Check sheet for the modelled part. Datum: model origin and axes. Units: mm. Face numbers are marked on the shaded views. Round coordinates to 2 decimals unless told otherwise and drop trailing zeros. Order: outer loops, then holes, each group sorted by start corner. A loop starts at its lowest first (then second) coordinate and runs counter-clockwise, first axis right, second up. Notation, with made-up numbers: (2.25, 18) -> (57.25, 18) arc R23 cw to (57.25, 38) -> close; hole circle Ø7 at (21.25, -16.5). An arc over 180 degrees is marked (long way). Answer as CSV lines item,"result". Start each with the question number.
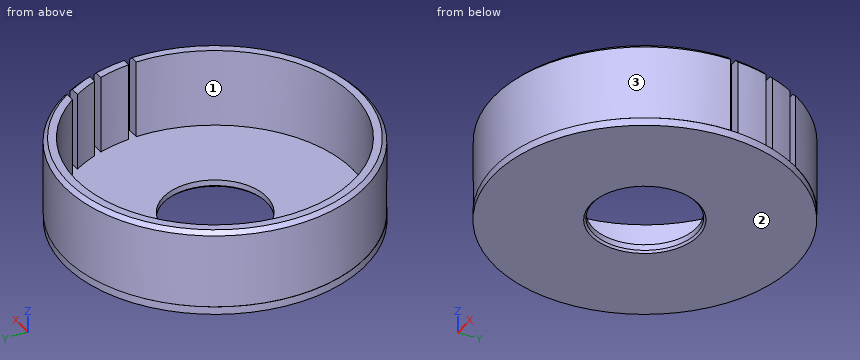
from build123d import *

# Parameters (mm, degrees)
SKETCH_R        = 38.5
SKETCH_R_2      = 13.2
PAD_DEPTH       = 2
PAD001_DEPTH    = 20
PAD002_DEPTH    = 20
PAD003_DEPTH    = 20
CHAMFER_SIZE    = 1
CHAMFER001_SIZE = 1
CHAMFER002_SIZE = 1
CHAMFER003_SIZE = 0.5


with BuildPart() as part:
    # Sketch → Pad (new body)
    with BuildSketch(Plane.XY):
        Circle(SKETCH_R)
        Circle(SKETCH_R_2, mode=Mode.SUBTRACT)
    extrude(amount=PAD_DEPTH)

    # Sketch001 (on Face4 of Pad) → Pad001 (join)
    with BuildSketch(Plane.XY.offset(2)):
        with BuildLine():
            ThreePointArc((29.4355806661, 19.9653668161), (-33.881351172, -10.373953904), (35.5584664799, 5.03191e-05))
            Line((35.5584664799, 5.03191e-05), (38.5584677887, 5.03191e-05))
            ThreePointArc((32.9980317105, 19.9653668161), (-37.0299944858, -10.2947354738), (38.5584677887, 5.03191e-05))
            Line((32.9980317105, 19.9653668161), (29.4355806661, 19.9653668161))
        make_face()
    extrude(amount=PAD001_DEPTH)

    # Sketch002 (on Face4 of Pad001) → Pad002 (join)
    with BuildSketch(Plane.XY.offset(2)):
        with BuildLine():
            ThreePointArc((38.4481958149, 1.9965566804), (38.0259798013, 6.0228614586), (37.1833064686, 9.9825708144))
            Line((37.1833064686, 9.9825708144), (34.0675546515, 9.9825708144))
            ThreePointArc((35.4438113275, 1.9965566804), (34.9843051311, 6.02896297), (34.0675546515, 9.9825708144))
            Line((35.4438113275, 1.9965566804), (38.4481958149, 1.9965566804))
        make_face()
    extrude(amount=PAD002_DEPTH)

    # Sketch003 (on Face3 of Pad002) → Pad003 (join)
    with BuildSketch(Plane.XY.offset(2)):
        with BuildLine():
            Line((33.4177914057, 11.9791993709), (36.5889161145, 11.9791993709))
            ThreePointArc((36.5889161145, 11.9791993709), (35.4459881583, 15.0277051968), (34.0495834936, 17.9687468653))
            Line((34.0495834936, 17.9687468653), (30.6165663668, 17.9687468653))
            ThreePointArc((33.4177914057, 11.9791993709), (32.1569341454, 15.0393346386), (30.6165663668, 17.9687468653))
        make_face()
    extrude(amount=PAD003_DEPTH)

    # Chamfer
    chamfer_edges = [part.edges().sort_by_distance(p)[0] for p in [
        (-37.029994, -10.294735, 22),
    ]]
    chamfer(chamfer_edges, length=CHAMFER_SIZE)

    # Chamfer001
    chamfer001_edges = [part.edges().sort_by_distance(p)[0] for p in [
        (38.02598, 6.022861, 22),
    ]]
    chamfer(chamfer001_edges, length=CHAMFER001_SIZE)

    # Chamfer002
    chamfer002_edges = [part.edges().sort_by_distance(p)[0] for p in [
        (35.445988, 15.027705, 22),
    ]]
    chamfer(chamfer002_edges, length=CHAMFER002_SIZE)

    # Chamfer003
    chamfer003_edges = [part.edges().sort_by_distance(p)[0] for p in [
        (-13.2, 0, 0),
    ]]
    chamfer(chamfer003_edges, length=CHAMFER003_SIZE)


solid = part.part
1) Material ranges on line 1 along Y through (x, z) = (0, 1.25); line 2 along Y through (x, z) = (31, 10.25); line 3 along Z through (x, y) = (0, 26.5), recorded low to high.
2) Depth check by flat-ended pin: pin 1 Ø2.5 at (x, z) = (33, 10) entering from +Y; pin 2 Ø8 at (y, z) = (-5, 16.5) entering from -X; pin 3 Ø12 at (x, z) = (18.5, 17) entering from +Y. Enter the tip coordinate at first touch or a pass-through.
3) Mould release check, pull along Y, two halves, no side actions. Record for the marked faces 1, 2 and 3: released by +Y, released by -Y, zero draft, split by the parting line, or undercut.
4) Section check A-A on z = 18.5. Record the cut outline in (x, y).
Solutions:
1,line 1,"y = -38.5 to -13.2, 13.2 to 38.5"
1,line 2,"y = -22.88 to -17.37, 17.3 to 17.97, 19.97 to 22.94"
1,line 3,"z = 0 to 2"
2,pin 1,"stops at y = 21.9"
2,pin 2,"stops at x = -38.43"
2,pin 3,"stops at y = 36.47"
3,face 1,"undercut"
3,face 2,"zero draft"
3,face 3,"split by the parting line"
4,outline,"(29.44, 19.97) -> (33, 19.97) arc R38.5 ccw (long way) to (38.56, 0) -> (35.56, 0) arc R35.5 cw (long way) to start; (30.62, 17.97) arc R35.5 cw to (33.42, 11.98) -> (36.59, 11.98) arc R38.5 ccw to (34.05, 17.97) -> close; (34.07, 9.98) arc R35.5 cw to (35.44, 2) -> (38.45, 2) arc R38.5 ccw to (37.18, 9.98) -> close"
